Can you work these out from the model? Positions are in its coordinate system, mm. Face numbers are marked on the shaded views. A direction names the side the tool comes from. Coordinates: 2 decimals unless noted, no trailing zeros. Order: outer loops, then holes, each group sorted by start corner. A loop starts at its lowest first (then second) coordinate and runs counter-clockwise, first axis right, second up. Notation, with made-up numbers: (88, 65.25) -> (140, 65.25) arc R27 ccw to (140, 100.25) -> close; hole circle Ø10 at (-7, -22). An arc over 180 degrees is marked (long way). Answer as a JSON object with one key per item and string values. Group by question number.
(1) Which directions (+Z, -Z, +X, -X, +Y, -Y) give clear straight access to the entire face, cutting with the end or side of a thin tool? Please do the marked faces 4, 5 and 6.
(2) I need wall thicknesses on line 1 (Z direction, x = 40, y = -60); line 2 (Z direction, x = 0, y = -24) (1 decimal); line 3 (Z direction, x = 67, y = -19). Which ranges of each line are inside material? Lowest first, please.
(3) I want a section at A-A, the plane y = -33. State how many separate pieces and enclosed holes the cut face has, plus the area to 3 significant figures.
(4) For pin 1 (3 mm diameter, centred on x = 15, y = -29.5, fed in from -Z); pin 2 (4 mm diameter, centred on y = -27, z = 31, fed in from -X); pin 3 (9 mm diameter, centred on x = 50.69, y = -12.7, fed in from -Z); pin 4 (1 mm diameter, centred on y = -30.5, z = -9, fed in from -X), each with a flat end and sliding along its axis, tell me the tip position at first contact or that it passes through.
(5) If we mould it in two halves opening along Y, with no side actions, what happens to the marked faces 1, 2 and 3? For each: pulls with the +Y half, pulls with the -Y half, needs draft (parallel to the pull), parting line crosses it, or undercut.
(6) I want a section at B-B, the plane z = -12.5. List the corners of the cut face in (x, y) for me, plus the area to 3 significant figures.
from build123d import *

# Parameters (mm, degrees)
F0_R     = 14.2875
F1_DEPTH = 63.5
F3_START = 28.40385
F2_R     = 5.5626
F3_DEPTH = 4.94635
F4_R     = 5.5626
F5_DEPTH = 33.3512


with BuildPart() as f1:
    # F0 (on Front) → F1 (new body)
    with BuildSketch(Plane.XZ):
        with BuildLine():
            Line((37.9924699664, 28.575), (0, 28.575))
            ThreePointArc((0, 28.575), (-20.2055762724, -20.2055762724), (28.575, 0))
            Line((28.575, 0), (28.575, 3.175))
            ThreePointArc((28.575, 3.175), (31.3648079092, 9.9101920908), (38.1, 12.7))
            Line((38.1, 12.7), (69.85, 12.7))
            Line((69.85, 12.7), (95.0348461551, 12.7))
            Line((95.0348461551, 12.7), (95.0348461551, 33.3502))
            Line((95.0348461551, 33.3502), (37.9924699664, 33.3502))
            Line((37.9924699664, 33.3502), (37.9924699664, 28.575))
        make_face()
        Circle(F0_R, mode=Mode.SUBTRACT)
    extrude(amount=F1_DEPTH)

    # F2 (on Top) → F3 (cut)
    with BuildSketch(Plane.XY.offset(F3_START)):
        with BuildLine():
            ThreePointArc((37.9924699664, -12.7), (41.6741160957, -3.757548703), (50.5849399165, 0))
            Line((50.5849399165, 0), (37.9924699664, 0))
            Line((37.9924699664, 0), (37.9924699664, -12.7))
        make_face()
        with BuildLine():
            Line((50.5849399165, 0), (50.8, 0))
            ThreePointArc((50.8, 0), (50.6924699583, 0.000455233), (50.5849399165, 0))
        make_face()
        with BuildLine():
            Line((37.9924699664, -63.5), (50.2103307418, -63.5))
            ThreePointArc((50.2103307418, -63.5), (42.2169815898, -60.4261048405), (37.9924699664, -52.9765435338))
            Line((37.9924699664, -52.9765435338), (37.9924699664, -63.5))
        make_face()
        with BuildLine():
            ThreePointArc((50.2103307418, -63.5), (50.5051653709, -63.5034228021), (50.8, -63.5))
            Line((50.8, -63.5), (50.2103307418, -63.5))
        make_face()
        with Locations((84.1502, -31.75)):
            Circle(F2_R)
        with Locations((50.6924699583, -12.699544767)):
            Circle(F2_R)
        with Locations((50.5051653709, -50.8034228021)):
            Circle(F2_R)
    extrude(amount=F3_DEPTH, mode=Mode.SUBTRACT)

    # F4 (on Top) → F5 (cut, through all)
    with BuildSketch(Plane.XY):
        with BuildLine():
            Line((84.0428003407, -48.5551651302), (50.6926003407, -63.5))
            Line((50.6926003407, -63.5), (95.0348461551, -63.5))
            Line((95.0348461551, -63.5), (95.0348461551, 0))
            Line((95.0348461551, 0), (50.6926003407, 0.0004552323))
            Line((50.6926003407, 0.0004552323), (84.0428003407, -14.9443796375))
            ThreePointArc((84.0428003407, -14.9443796375), (94.9275939219, -31.7497723839), (84.0428003407, -48.5551651302))
        make_face()
        with Locations((84.0428003407, -31.7497723839)):
            Circle(F4_R)
        with Locations((50.6924699583, -12.699544767)):
            Circle(F4_R)
        with Locations((50.6926003407, -50.8)):
            Circle(F4_R)
    extrude(amount=F5_DEPTH, mode=Mode.SUBTRACT)


solid = f1.part
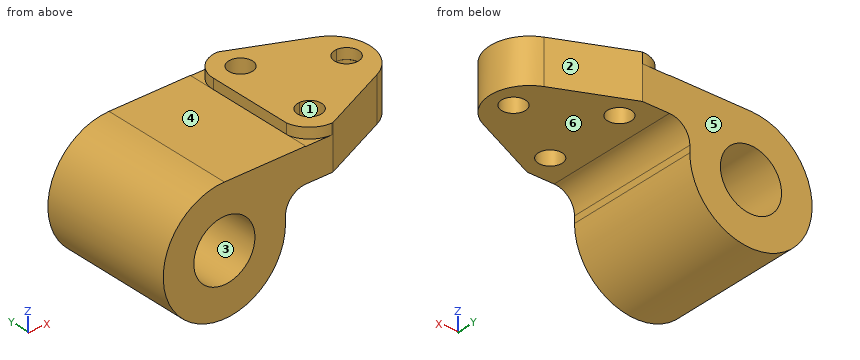
Computed values:
{
 "1": {"face 4": "+Z, -X, +Y, -Y", "face 5": "+Z, -Z, +X, -X, +Y", "face 6": "-Z, +X, +Y, -Y"},
 "2": {"line 1": "z = 12.7 to 28.4", "line 2": "z = -28.6 to -14.3, 14.3 to 28.6", "line 3": "z = 12.7 to 33.35"},
 "3": {"separate pieces": "2", "enclosed holes": "1", "area": "3,220 mm2"},
 "4": {"pin 1": "stops at z = -25.18", "pin 2": "stops at x = 37.99", "pin 3": "passes through", "pin 4": "stops at x = -27.28"},
 "5": {"face 1": "undercut", "face 2": "pulls with the +Y half", "face 3": "needs draft"},
 "6": {"outline": "(-25.7, -63.5) -> (-6.92, -63.5) -> (-6.92, 0) -> (-25.7, 0) -> close; (6.92, -63.5) -> (25.7, -63.5) -> (25.7, 0) -> (6.92, 0) -> close", "area": "2,380 mm2"}
}
